Part model, mm, in its own coordinate system. A direction names the side the tool comes from. Coordinates: 2 decimals unless noted, no trailing zeros. Write each loop counter-clockwise with the first axis right and the second up, starting at its lowest first coordinate (ties: lowest second). Pieces come first, ordered by that corner, then holes. Notation, with made-up numbers: (-38, 54.25) -> (2, 54.25) arc R29 cw to (2, 74.25) -> close; hole circle Ø7 at (66, -15). An arc over 180 degrees is marked (long way). Write item = value, one per line. Start each with the question number.
Q1. Band-saw the part on A-A, the plane y = 63. List the corners of the cut face in (x, z) (1 decimal), plus the area to 3 significant figures.
Q2. Probe line 1 (X direction, y = 10, z = -1); line 2 (Y direction, x = 0, z = -2); line 3 (Z direction, x = 51.5, y = 56.5) (3 decimals). List the from-to ranges inside material, lowest first.
Q3. Tool access for faces 4 (the cylindrical face through (133.232, -3.423, -1.984)), 5 (the flat face through (10, 28, -2)), 6 (the flat face through (133, 6, 7.88)): list every direction of +Z, -Z, +X, -X, +Y, -Y with a clear straight run to the whole face (end or side of a thin tool).
Q4. Pull direction Y, two halves, no side cores. Call faces 1 (the cylindrical face through (-4.6, 118.88, -1.61)), 2 (the cylindrical face through (135.753, 11.322, 9.445)), 3 (the flat face through (133, -4.678, 4)): released by +Y, released by -Y, zero draft, split by the parting line, or undercut.
Q5. Band-saw the part on D-D, the plane x = 16. List the corners of the cut face in (y, z) (1 decimal).
Q6. Pin check, flat tips, straight feed: P1, Ø3, axis at x = 39.5, y = 68, coming from the -Z side (3 decimals); P2, Ø6.5, axis at x = 130, z = 5, coming from the -Y side; P3, Ø3, axis at y = 61, z = 0, coming from the +X side; P4, Ø7, axis at x = 133.37, y = 9.5, coming from the +Z side (3 decimals). Stop position of each tip, or through.
Q7. Band-saw the part on B-B, the plane z = 5. List the corners of the cut face in (x, y), plus the area to 3 significant figures.
Q8. Band-saw the part on C-C, the plane x = 0. Give the number of separate pieces and of enclosed holes in the cut face, plus the area to 3 significant figures.
from build123d import *

# Parameters (mm, degrees)
BASE_FLANGE1_DEPTH           = 3.175
EDGE_FLANGE3_DEPTH           = 20
EDGE_FLANGE4_STRIP_W         = 14.7
EDGE_FLANGE4_STRIP_H         = 3.175
EDGE_FLANGE4_STRIP_CUT_DEPTH = 20
EDGE_FLANGE4_DEPTH           = 20
CUT_EXTRUDE1_DEPTH           = 194.888053308
CUT_EXTRUDE1_DEPTH_BACK      = 194.888053308
SKETCH12_R                   = 3
TAB1_DEPTH                   = 3.175
EDGE_FLANGE5_DEPTH           = 20.110165591
FILLET1_R                    = 10
FILLET2_R                    = 5
SKETCH27_R                   = 2.155423697
CUT_EXTRUDE2_DEPTH           = 196.8016212


# Sheet-metal steps are written as plain solids
with BuildPart() as part:
    # Sketch1 → Base-Flange1 (new body)
    with BuildSketch(Plane.XY):
        Polygon((10, 0), (10, 84.928918998), (123.372130178, -0.503108866), (143.372130178, -0.503108866), (143.372130178, 14.482707214), (-10, 130.056897083), (-10, 0), align=None)
    extrude(amount=-BASE_FLANGE1_DEPTH)

    # Edge-Flange3 section (across the edge) → Edge-Flange3 (add)
    with BuildSketch(Plane(origin=(123.372130178, -1.503108866, 0), x_dir=(0, 1, 0), z_dir=(1, 0, 0))):
        with BuildLine():
            Line((-3.175, 1), (-3.175, 11.055))
            Line((-3.175, 11.055), (0, 11.055))
            Line((0, 11.055), (0, 1))
            ThreePointArc((0, 1), (0.292893219, 0.292893219), (1, 0))
            Line((1, 0), (1, -3.175))
            ThreePointArc((1, -3.175), (-1.952170811, -1.952170811), (-3.175, 1))
        make_face()
    extrude(amount=EDGE_FLANGE3_DEPTH)

    # Edge-Flange4 strip (across the edge) → Edge-Flange4 strip cut (cut)
    with BuildSketch(Plane(origin=(123.372130178, -1.503108866, 11.055), x_dir=(0, 0, -1), z_dir=(1, 0, 0))):
        with Locations((-3.175, -1.5875)):
            Rectangle(EDGE_FLANGE4_STRIP_W, EDGE_FLANGE4_STRIP_H)
    extrude(amount=EDGE_FLANGE4_STRIP_CUT_DEPTH, mode=Mode.SUBTRACT)

    # Edge-Flange4 section (across the edge) → Edge-Flange4 (add)
    with BuildSketch(Plane(origin=(123.372130178, -1.503108866, 11.055), x_dir=(0, 0, -1), z_dir=(1, 0, 0))):
        with BuildLine():
            Line((0, 1), (0, 16.825))
            Line((0, 16.825), (3.175, 16.825))
            Line((3.175, 16.825), (3.175, 1))
            ThreePointArc((3.175, 1), (3.467893219, 0.292893219), (4.175, 0))
            Line((4.175, 0), (4.175, -3.175))
            ThreePointArc((4.175, -3.175), (1.222829189, -1.952170811), (0, 1))
        make_face()
    extrude(amount=EDGE_FLANGE4_DEPTH)

    # Sketch12 → Cut-Extrude1 (cut, two sides: drawn at the far end of the back side and taken through both)
    with BuildSketch(Plane.XY.offset(-CUT_EXTRUDE1_DEPTH_BACK)):
        with Locations(Location((133.372130178, 9.496891134, 0), (0, 0, 180))):
            Circle(SKETCH12_R)
        with Locations((0, 10)):
            Circle(SKETCH12_R)
    extrude(amount=CUT_EXTRUDE1_DEPTH + CUT_EXTRUDE1_DEPTH_BACK, mode=Mode.SUBTRACT)

    # Sketch19 → Tab1 (add)
    with BuildSketch(Plane.XY):
        Polygon((-10, 0), (10, 0), (10, -10), (-10, -7.897915295), align=None)
    extrude(amount=-TAB1_DEPTH)

    # Edge-Flange5 section (across the edge) → Edge-Flange5 (add)
    with BuildSketch(Plane(origin=(9.895471537, -10.994521895, -3.175), x_dir=(0.10452846326765029, 0.9945218953682737, -3.4914813388431334e-15), z_dir=(-0.9945218953682737, 0.10452846326765029, 0))):
        with BuildLine():
            Line((-3.175, 1), (-3.175, 21.825))
            Line((-3.175, 21.825), (0, 21.825))
            Line((0, 21.825), (0, 1))
            ThreePointArc((0, 1), (0.292893219, 0.292893219), (1, 0))
            Line((1, 0), (1, -3.175))
            ThreePointArc((1, -3.175), (-1.952170811, -1.952170811), (-3.175, 1))
        make_face()
    extrude(amount=EDGE_FLANGE5_DEPTH)

    # Fillet1
    fillet1_edges = [part.edges().sort_by_distance(p)[0] for p in [
        (-10, 130.056897083, -1.5875),
        (10, 84.928918998, -1.5875),
    ]]
    fillet(fillet1_edges, radius=FILLET1_R)

    # Fillet2
    fillet2_edges = [part.edges().sort_by_distance(p)[0] for p in [
        (9.729532601, -12.573325404, -25),
        (-10.270467399, -10.471240699, -25),
        (143.372130178, 14.482707214, -1.5875),
        (123.372130178, 15.321891134, 9.4675),
        (143.372130178, 15.321891134, 9.4675),
    ]]
    fillet(fillet2_edges, radius=FILLET2_R)

    # Sketch27 → Cut-Extrude2 (cut, through all)
    with BuildSketch(Plane(origin=(-1.034824921, -9.845701445, 0), x_dir=(0.9945218953682736, -0.10452846326765024, 0), z_dir=(0.10452846326765025, 0.9945218953682737, -3.503032532656101e-15))):
        with Locations(Location((0.935420791, 20, 0), (0, 0, 180))):
            Circle(SKETCH27_R)
        with Locations(Location((0.935420791, 10, 0), (0, 0, 180))):
            Circle(SKETCH27_R)
    extrude(amount=-CUT_EXTRUDE2_DEPTH, mode=Mode.SUBTRACT)


solid = part.part
Ans:
q1.outline = (-10, -3.2) -> (10, -3.2) -> (10, 0) -> (-10, 0) -> close; (39.1, -3.2) -> (79, -3.2) -> (79, 0) -> (39.1, 0) -> close
q1.area = 190 mm2
q2.line_1 = -10 to -3, 3 to 10, 109.43 to 130.41, 136.33 to 143.37
q2.line_2 = -12.53 to 7, 13 to 120
q2.line_3 = -3.175 to 0
q3.face_4 = -Z, +X, -Y
q3.face_5 = +Z, -Z, -Y
q3.face_6 = +X, -X, +Y
q4.face_1 = released by +Y
q4.face_2 = undercut
q4.face_3 = released by -Y
q5.outline = (74, -3.2) -> (110.5, -3.2) -> (110.5, 0) -> (74, 0) -> close
q6.P1 = -3.175
q6.P2 = -4.68
q6.P3 = 83.63
q6.P4 = 11.055
q7.outline = (123.37, -4.68) -> (143.37, -4.68) -> (143.37, -1.5) -> (123.37, -1.5) -> close
q7.area = 63.5 mm2
q8.separate_pieces = 4
q8.enclosed_holes = 0
q8.area = 443 mm2
